Geometry check sheet. Reference: drawing and pictorial views, mm from the part's lowest x, y, z. Coordinates: 2 decimals unless noted, no trailing zeros. Write each loop counter-clockwise with the first axis right and the second up, starting at its lowest first coordinate (ties: lowest second). Pieces come first, ordered by that corner, then holes. Notation, with made-up numbers: (-13.5, 50.25) - (14.5, 50.25) arc R15 cw to (14.5, 57.25) - close; hole circle Ø5 at (18.25, -12). An arc over 180 degrees is marked (long way). Use one line per item in the form item = value. Start each with the question number.
(1) Material ranges on line 1 (X direction, y = 0.45, z = 5.5) (1 decimal); line 2 (X direction, y = 1.45, z = 4.75) (1 decimal); line 3 (X direction, y = 0.7, z = 8), recorded low to high. Write a range as [from, to].
(2) Gauge pin test, flat end, axial feed: pin 1 Ø1 at (y, z) = (0.5, 1.5) entering from -X (1 decimal). Record the tip position at first contact, or that the pin passes through.
(3) Mould release check, pull along Y, two halves, no side actions. Record for the marked faces 1 and 2: released by +Y, released by -Y, zero draft, split by the parting line, or undercut.
(4) Sectioned sample at A-A (y = 1.25). Record the cut outline in (x, z) (1 decimal), and give its area (3 significant figures).
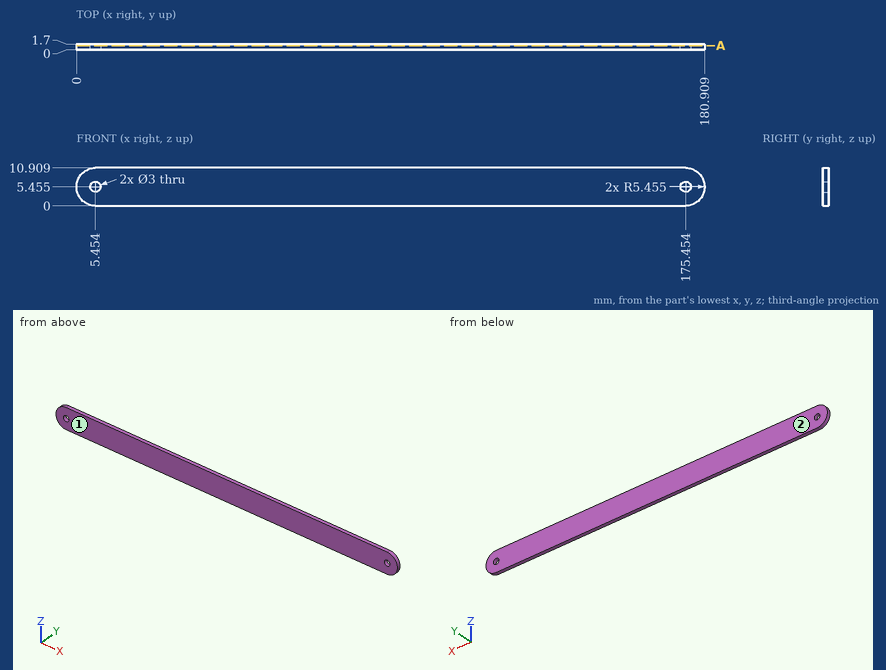
Answers below:
q1.line_1 = [0, 4], [7, 174], [177, 180.9]
q1.line_2 = [0, 4.1], [6.8, 174.1], [176.8, 180.9]
q1.line_3 = [0.63, 180.28]
q2.pin_1 = 1.2
q3.face_1 = released by -Y
q3.face_2 = released by +Y
q4.outline = (5.5, 0) - (175.5, 0) arc R5.5 ccw to (175.5, 10.9) - (5.5, 10.9) arc R5.5 ccw to start; hole circle Ø3 at (5.5, 5.5); hole circle Ø3 at (175.5, 5.5)
q4.area = 1,930 mm2
